Read the model definition and answer for the solid it produces. Units are mm, in the model's axes. Face numbers are marked on the shaded views. A direction names the side the tool comes from. Round coordinates to 2 decimals unless told otherwise and drop trailing zeros. Write each loop counter-clockwise with the first axis right and the second up, starting at its lowest first coordinate (ties: lowest second). Pieces come first, ordered by that corner, then holes. Notation, with made-up numbers: (-27, 87.5) -> (13, 87.5) arc R30 cw to (13, 125.5) -> close; hole circle Ø11 at (-34, 78). An arc over 180 degrees is marked (long way). Return JSON: item names as keys, results as strings. Group by question number.
(1) Straight lines are drawn through the part: line 1 (Y direction, x = 80, z = 3.75); line 2 (X direction, y = -44, z = 2.5); line 3 (Y direction, x = 82.5, z = 7.5). For each, find the intervals that lie inside material, in ascending order.
(2) A cutting plane is placed at C-C on x = 90. Give the vertices of the cut face in (y, z).
(3) A cutting plane is placed at D-D on z = 3.5. Give the vertices of the cut face in (x, y), then the cut area to 3 significant figures.
(4) For the marked faces 1 and 2, determine the directions among +Z, -Z, +X, -X, +Y, -Y from which every point of the face is accessible in a straight line to the end or side of a thin tool.
(5) The mould has two halves that part along Y. Classify the marked faces 3, 4 and 5: released by +Y, released by -Y, zero draft, split by the parting line, or undercut.
(6) A cutting plane is placed at B-B on y = -39.5. Give the vertices of the cut face in (x, z).
(7) A cutting plane is placed at A-A on x = 77.25. Give the vertices of the cut face in (y, z).
```python
from build123d import *

# Parameters (mm, degrees)
SKETCH_1_W          = 100
SKETCH_1_H          = 100
EXTRUDE_1_DEPTH     = 8
SKETCH_2_R          = 2.15
CUT_EXTRUDE_1_DEPTH = 142.647449677
SKETCH_3_R          = 2.15
CUT_EXTRUDE_2_DEPTH = 142.647449677
SKETCH_4_R          = 2.15
CUT_EXTRUDE_3_DEPTH = 142.647449677
SKETCH_5_W          = 20.5
SKETCH_5_H          = 41.5
CUT_EXTRUDE_4_DEPTH = 10
SKETCH_6_W          = 55
SKETCH_6_H          = 100
CUT_EXTRUDE_5_DEPTH = 10
FILLET_2_R          = 1.2
SKETCH_8_R          = 1.65
CUT_EXTRUDE_6_DEPTH = 142.647449677
SKETCH_9_W          = 15.75
SKETCH_9_H          = 78.5
CUT_EXTRUDE_7_DEPTH = 142.647449677
FILLET_3_R          = 10
FILLET_4_R          = 3
SKETCH_10_R         = 1.65
SKETCH_10_R_2       = 2.15
CUT_EXTRUDE_8_DEPTH = 142.647449677
FILLET_5_R          = 3


with BuildPart() as part:
    # 草图1 → 凸台-拉伸1 (new body)
    with BuildSketch(Plane.XY):
        with Locations((50, -50)):
            Rectangle(SKETCH_1_W, SKETCH_1_H)
    extrude(amount=EXTRUDE_1_DEPTH)

    # 草图2 → 切除-拉伸1 (cut, through all)
    with BuildSketch(Plane.XY.offset(8)):
        with Locations((80, -53)):
            Circle(SKETCH_2_R)
        with Locations((90, -53)):
            Circle(SKETCH_2_R)
        with Locations((90, -5)):
            Circle(SKETCH_2_R)
        with Locations((80, -5)):
            Circle(SKETCH_2_R)
    extrude(amount=-CUT_EXTRUDE_1_DEPTH, mode=Mode.SUBTRACT)

    # 草图3 → 切除-拉伸2 (cut, through all)
    with BuildSketch(Plane.XY.offset(8)):
        with Locations((73, -95)):
            Circle(SKETCH_3_R)
        with Locations((73, -85)):
            Circle(SKETCH_3_R)
        with Locations((85, -85)):
            Circle(SKETCH_3_R)
        with Locations((85, -95)):
            Circle(SKETCH_3_R)
    extrude(amount=-CUT_EXTRUDE_2_DEPTH, mode=Mode.SUBTRACT)

    # 草图4 → 切除-拉伸3 (cut, through all)
    with BuildSketch(Plane.XY.offset(8)):
        with BuildLine():
            ThreePointArc((81, -100), (71.5, -90.5), (62, -100))
            Line((62, -100), (81, -100))
        make_face()
        with Locations((73, -95)):
            Circle(SKETCH_4_R, mode=Mode.SUBTRACT)
    extrude(amount=-CUT_EXTRUDE_3_DEPTH, mode=Mode.SUBTRACT)

    # 草图5 → 切除-拉伸4 (cut)
    with BuildSketch(Plane.XY.offset(8)):
        with Locations((85, -29)):
            Rectangle(SKETCH_5_W, SKETCH_5_H)
    extrude(amount=-CUT_EXTRUDE_4_DEPTH, mode=Mode.SUBTRACT)

    # 草图6 → 切除-拉伸5 (cut)
    with BuildSketch(Plane.XY.offset(8)):
        with Locations((27.5, -50)):
            Rectangle(SKETCH_6_W, SKETCH_6_H)
    extrude(amount=-CUT_EXTRUDE_5_DEPTH, mode=Mode.SUBTRACT)

    # 圆角2
    fillet_2_edges = [part.edges().sort_by_distance(p)[0] for p in [
        (95.25, -49.75, 4),
        (74.75, -49.75, 4),
        (74.75, -8.25, 4),
        (95.25, -8.25, 4),
    ]]
    fillet(fillet_2_edges, radius=FILLET_2_R)

    # 草图8 → 切除-拉伸6 (cut, through all)
    with BuildSketch(Plane.XY.offset(8)):
        with Locations((59, -84)):
            Circle(SKETCH_8_R)
    extrude(amount=-CUT_EXTRUDE_6_DEPTH, mode=Mode.SUBTRACT)

    # 草图9 → 切除-拉伸7 (cut, through all)
    with BuildSketch(Plane.XY.offset(8)):
        with BuildLine():
            Line((71.5, -90.5), (55, -90.5))
            Line((55, -90.5), (55, -100))
            Line((55, -100), (62, -100))
            ThreePointArc((62, -100), (64.782485579, -93.282485579), (71.5, -90.5))
        make_face()
        with Locations((62.875, -39.25)):
            Rectangle(SKETCH_9_W, SKETCH_9_H)
    extrude(amount=-CUT_EXTRUDE_7_DEPTH, mode=Mode.SUBTRACT)

    # 圆角3
    fillet_3_edges = [part.edges().sort_by_distance(p)[0] for p in [
        (70.75, -78.5, 4),
    ]]
    fillet(fillet_3_edges, radius=FILLET_3_R)

    # 圆角4
    fillet_4_edges = [part.edges().sort_by_distance(p)[0] for p in [
        (55, -90.5, 4),
        (55, -78.5, 4),
        (70.75, 0, 4),
        (81, -100, 4),
        (100, 0, 4),
        (100, -100, 4),
    ]]
    fillet(fillet_4_edges, radius=FILLET_4_R)

    # 草图10 → 切除-拉伸8 (cut, through all)
    with BuildSketch(Plane.XY.offset(8)):
        with BuildLine():
            Line((100, -57), (70.75, -57))
            Line((70.75, -57), (70.75, -68.5))
            ThreePointArc((70.75, -68.5), (67.821067812, -75.571067812), (60.75, -78.5))
            Line((60.75, -78.5), (58, -78.5))
            ThreePointArc((58, -78.5), (55.878679656, -79.378679656), (55, -81.5))
            Line((55, -81.5), (55, -87.5))
            ThreePointArc((55, -87.5), (55.878679656, -89.621320344), (58, -90.5))
            Line((58, -90.5), (71.5, -90.5))
            ThreePointArc((71.5, -90.5), (77.356193303, -92.51969252), (80.722342436, -97.72))
            ThreePointArc((80.722342436, -97.72), (81.785336899, -99.362202362), (83.6346611, -100))
            Line((83.6346611, -100), (97, -100))
            ThreePointArc((97, -100), (99.121320344, -99.121320344), (100, -97))
            Line((100, -97), (100, -57))
        make_face()
        with Locations((59, -84)):
            Circle(SKETCH_10_R, mode=Mode.SUBTRACT)
        with Locations((73, -85)):
            Circle(SKETCH_10_R_2, mode=Mode.SUBTRACT)
        with Locations((85, -95)):
            Circle(SKETCH_10_R_2, mode=Mode.SUBTRACT)
        with Locations((85, -85)):
            Circle(SKETCH_10_R_2, mode=Mode.SUBTRACT)
    extrude(amount=-CUT_EXTRUDE_8_DEPTH, mode=Mode.SUBTRACT)

    # 圆角5
    fillet_5_edges = [part.edges().sort_by_distance(p)[0] for p in [
        (70.75, -57, 4),
        (100, -57, 4),
    ]]
    fillet(fillet_5_edges, radius=FILLET_5_R)


solid = part.part
```
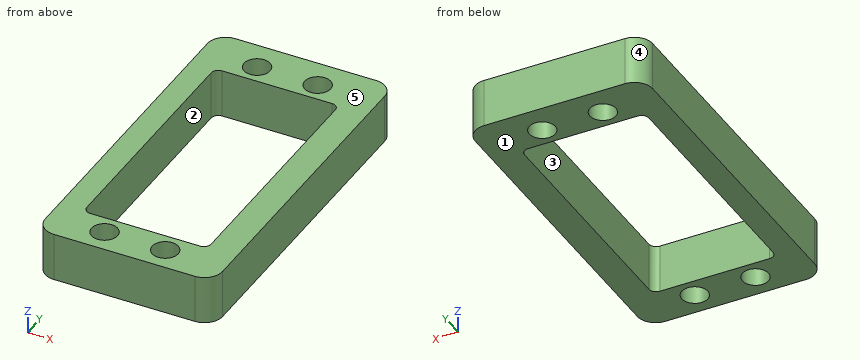
Checks:
{
 "1": {"line 1": "y = -57 to -55.15, -50.85 to -49.75, -8.25 to -7.15, -2.85 to 0", "line 2": "x = 70.75 to 74.75, 95.25 to 100", "line 3": "y = -57 to -49.75, -8.25 to 0"},
 "2": {"outline": "(-57, 0) -> (-55.15, 0) -> (-55.15, 8) -> (-57, 8) -> close; (-50.85, 0) -> (-49.75, 0) -> (-49.75, 8) -> (-50.85, 8) -> close; (-8.25, 0) -> (-7.15, 0) -> (-7.15, 8) -> (-8.25, 8) -> close; (-2.85, 0) -> (0, 0) -> (0, 8) -> (-2.85, 8) -> close"},
 "3": {"outline": "(70.75, -54) arc R3 ccw to (73.75, -57) -> (97, -57) arc R3 ccw to (100, -54) -> (100, -3) arc R3 ccw to (97, 0) -> (73.75, 0) arc R3 ccw to (70.75, -3) -> close; hole (74.75, -48.55) arc R1.2 ccw to (75.95, -49.75) -> (94.05, -49.75) arc R1.2 ccw to (95.25, -48.55) -> (95.25, -9.45) arc R1.2 ccw to (94.05, -8.25) -> (75.95, -8.25) arc R1.2 ccw to (74.75, -9.45) -> close; hole circle Ø4.3 at (80, -53); hole circle Ø4.3 at (80, -5); hole circle Ø4.3 at (90, -53); hole circle Ø4.3 at (90, -5)", "area": "752 mm^2"},
 "4": {"face 1": "-Z, +X, -X, +Y, -Y", "face 2": "+Z, -Z"},
 "5": {"face 3": "undercut", "face 4": "released by +Y", "face 5": "zero draft"},
 "6": {"outline": "(70.75, 0) -> (74.75, 0) -> (74.75, 8) -> (70.75, 8) -> close; (95.25, 0) -> (100, 0) -> (100, 8) -> (95.25, 8) -> close"},
 "7": {"outline": "(-57, 0) -> (-49.75, 0) -> (-49.75, 8) -> (-57, 8) -> close; (-8.25, 0) -> (0, 0) -> (0, 8) -> (-8.25, 8) -> close"}
}
